from build123d import *
from build123d.topology import SkipClean

# Parameters (mm, degrees)
REVOLVE1_ANGLE      = 5
CIRPATTERN1_COUNT   = 4
BOSS_EXTRUDE2_START = 160
SKETCH4_W           = 150
SKETCH4_H           = 100
BOSS_EXTRUDE2_DEPTH = 10


with BuildPart() as part:
    # Sketch1 → Revolve1 (revolve)
    with BuildSketch(Plane.XY):
        with BuildLine():
            Line((0, 165), (0, 155))
            ThreePointArc((0, 155), (-109.601551084, 109.601551084), (-155, 0))
            Line((-155, 0), (-165, 0))
            ThreePointArc((-165, 0), (-116.672618896, 116.672618896), (0, 165))
        make_face()
    revolve(axis=Axis((-165, 0, 0), (1, 0, 0)), revolution_arc=REVOLVE1_ANGLE)


with BuildPart() as cirpattern1_1:
    # CirPattern1: pattern copy
    add(part.part.rotate(Axis((0, 0, 0), (0, 1, 0)), 1 * 360 / CIRPATTERN1_COUNT))


with BuildPart() as cirpattern1_2:
    # CirPattern1: pattern copy
    add(part.part.rotate(Axis((0, 0, 0), (0, 1, 0)), 2 * 360 / CIRPATTERN1_COUNT))


with BuildPart() as cirpattern1_3:
    # CirPattern1: pattern copy
    add(part.part.rotate(Axis((0, 0, 0), (0, 1, 0)), 3 * 360 / CIRPATTERN1_COUNT))


with BuildPart() as part_1:
    with SkipClean():  # the faces are left unmerged after this step: merging them gives an invalid solid
        add(part.part)

        add(cirpattern1_1.part)  # Boss-Extrude2 merges CirPattern1_1

        add(cirpattern1_2.part)  # Boss-Extrude2 merges CirPattern1_2

        add(cirpattern1_3.part)  # Boss-Extrude2 merges CirPattern1_3
        # Sketch4 → Boss-Extrude2 (add)
        with BuildSketch(Plane(origin=(0, 0, 0), x_dir=(1, 0, 0), z_dir=(0, 1, 0)).offset(BOSS_EXTRUDE2_START)):
            Rectangle(SKETCH4_W, SKETCH4_H)
        extrude(amount=BOSS_EXTRUDE2_DEPTH)


solid = part_1.part
Build history of the part. All positions in model axes, mm. A direction names the side the tool comes from. Round coordinates to 2 decimals unless told otherwise and drop trailing zeros. Loops run counter-clockwise (first coordinate to the right, second up) from the corner with the lowest first, then second, coordinate; pieces in that order, holes last. Notation, with made-up numbers: (79, 81.5) -> (130, 81.5) arc R10 cw to (130, 87.5) -> close; hole circle Ø2 at (-16, -20). An arc over 180 degrees is marked (long way). Answer in a Markdown table with one row per item.
Item 1: Which spindle directions (+Z, -Z, +X, -X, +Y, -Y) get a long thin tool onto all of the face, cutting with end or side? Do faces 1 (the flat face through (0, 104, 117)), 2 (the flat face through (0, 104, -117)), 3 (the flat face through (-75, 165, 1)), 4 (the flat face through (117, 104, 0)). Say none if no direction does.
Answers below:
| item | result |
|---|---|
| face 1 | +Z, -X, -Y |
| face 2 | -Z, +X, -Y |
| face 3 | +Z, -Z, -X, +Y |
| face 4 | +Z, +X, -Y |
Item 2: Drill centre lines: L1, parallel to Y at x = 34, z = 41; L2, parallel to Z at x = 146.5, y = 66; L3, parallel to Y at x = -7, z = -31.5. Where is each one in solid material? Low to high. Write a range as [from, to].
Answers below:
| item | result |
|---|---|
| L1 | y = [160, 170] |
| L2 | z = [-5.77, 0] |
| L3 | y = [151.6, 170] |
Item 3: Saw through at D-D (y = 16). Write the cut outline in (x, z), and give its area (3 significant figures).
Answers below:
| item | result |
|---|---|
| outline | (-164.22, 0) -> (-154.17, 0) arc R154.17 cw to (-154.17, 1.4) -> (-164.22, 1.4) arc R164.22 ccw to start; (-1.4, -164.22) arc R164.22 ccw to (0, -164.22) -> (0, -154.17) arc R154.17 cw to (-1.4, -154.17) -> close; (0, 154.17) arc R154.17 cw to (1.4, 154.17) -> (1.4, 164.22) arc R164.22 ccw to (0, 164.22) -> close; (154.17, -1.4) -> (164.22, -1.4) arc R164.22 ccw to (164.22, 0) -> (154.17, 0) arc R154.17 cw to start |
| area | 56.3 mm² |
Item 4: Pin check, flat tips, straight feed: pin 1 (12 mm diameter, centred on y = 99.5, z = 120.5, fed in from -X); pin 2 (5 mm diameter, centred on y = 166.5, z = 1.5, fed in from +X); pin 3 (3 mm diameter, centred on x = 9, y = 166.5, fed in from -Z). Stop position of each tip, or through.
Answers below:
| item | result |
|---|---|
| pin 1 | stops at x = 0 |
| pin 2 | stops at x = 75 |
| pin 3 | stops at z = -50 |
Item 5: Saw through at C-C (z = -31.5). Write the cut outline in (x, y).
Answers below:
| item | result |
|---|---|
| outline | (-75, 160) -> (-14, 160) -> (-13.23, 151.19) arc R151.77 cw to (0, 151.77) -> (0, 160) -> (75, 160) -> (75, 170) -> (-75, 170) -> close |
Item 6: Saw through at A-A (y = 39). Write the cut outline in (x, z).
Answers below:
| item | result |
|---|---|
| outline | (-160.32, 0) -> (-150.01, 0) arc R150.01 cw to (-149.97, 3.41) -> (-160.29, 3.41) arc R160.32 ccw to start; (-3.41, -160.29) arc R160.32 ccw to (0, -160.32) -> (0, -150.01) arc R150.01 cw to (-3.41, -149.97) -> close; (0, 150.01) arc R150.01 cw to (3.41, 149.97) -> (3.41, 160.29) arc R160.32 ccw to (0, 160.32) -> close; (149.97, -3.41) -> (160.29, -3.41) arc R160.32 ccw to (160.32, 0) -> (150.01, 0) arc R150.01 cw to start |
Item 7: Saw through at B-B (x = 61.5). Write the cut outline in (y, z), and give its area (3 significant figures).
Answers below:
| item | result |
|---|---|
| outline | (141.74, -12.4) -> (152.53, -13.34) arc R153.11 ccw to (153.11, 0) -> (142.28, 0) arc R142.28 cw to start; (160, -50) -> (170, -50) -> (170, 50) -> (160, 50) -> close |
| area | 1,140 mm² |
